Study the drawing (mm; zero at the part's minimum x, y, z) and answer. Round coordinates to 2 decimals unless told otherwise and drop trailing zeros. Order: outer loops, then holes, each group sorted by start corner. A loop starts at its lowest first (then second) coordinate and runs counter-clockwise, first axis right, second up. Notation, with made-up numbers: M 10.25,-33.5 L 24.25,-33.5 A24 ccw 24.25,-17.5 Z; hole C 30.25,-6.75 d6. An arc over 180 degrees is marked long. Put each result on its own line as item: value. Start each with the question number.
1. The part is cut by section C-C (z = 133.5). Give the vertices of the cut face in (x, y), then the cut area to 3 significant figures.
2. Consider line 1 (Z direction, x = 28, y = 1.7); line 2 (Z direction, x = 24.5, y = 1.8); line 3 (X direction, y = 1.2, z = 138). Determine where each line is inside the solid, lowest interval first.
3. The part is cut by section B-B (x = 142). Give the vertices of the cut face in (y, z), then the cut area to 3 significant figures.
4. The part is cut by section A-A (y = 1.15). Give the vertices of the cut face in (x, z).
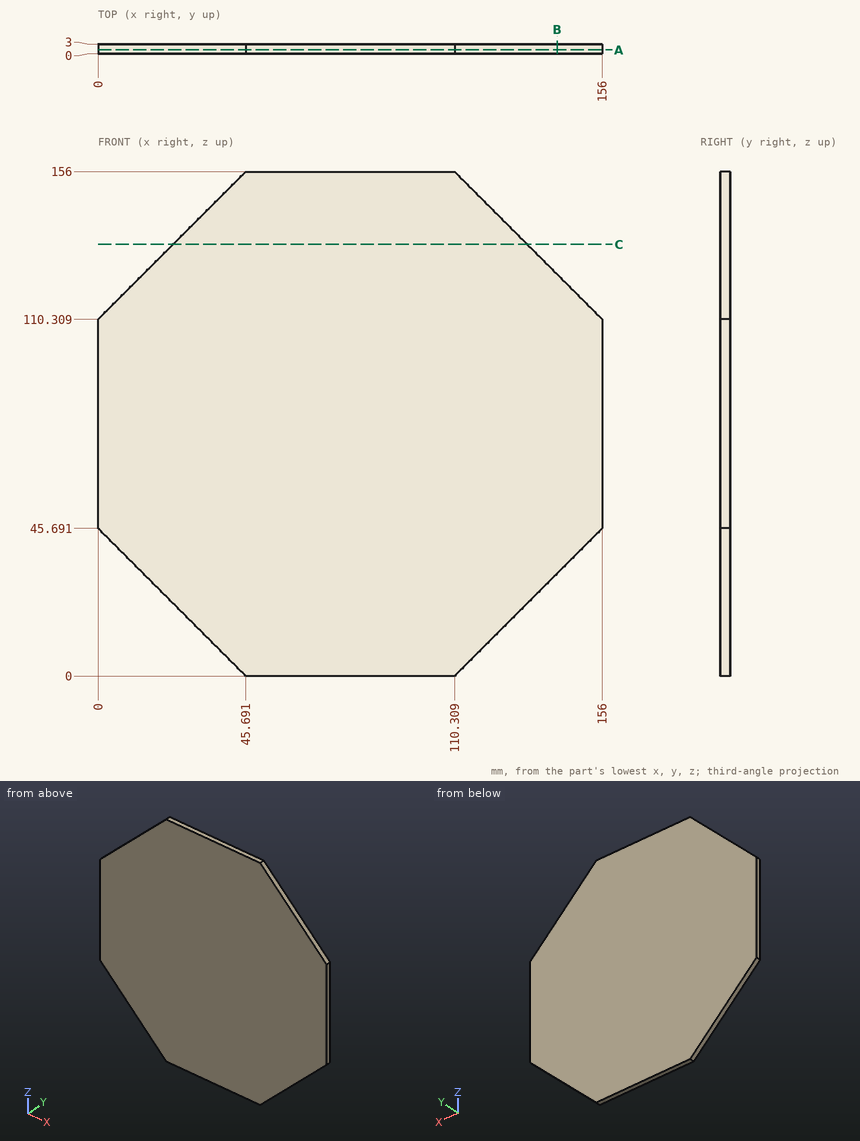
Resolved:
1. outline: M 23.19,0 L 132.81,0 L 132.81,3 L 23.19,3 Z
1. area: 329 mm2
2. line 1: 17.69 to 138.31
2. line 2: 21.19 to 134.81
2. line 3: 27.69 to 128.31
3. outline: M 0,31.69 L 3,31.69 L 3,124.31 L 0,124.31 Z
3. area: 278 mm2
4. outline: M 0,45.69 L 45.69,0 L 110.31,0 L 156,45.69 L 156,110.31 L 110.31,156 L 45.69,156 L 0,110.31 Z
